```python
from build123d import *

# Parameters (mm, degrees)
BOSS_EXTRUDE1_DEPTH = 480


with BuildPart() as part:
    # Sketch1 → Boss-Extrude1 (new body)
    with BuildSketch(Plane(origin=(0, 0, 0), x_dir=(1, 0, 0), z_dir=(0, 1, 0))):
        with BuildLine():
            Line((20, 5.42), (20, 0.5))
            ThreePointArc((20, 0.5), (19.853553391, 0.146446609), (19.5, 0))
            Line((19.5, 0), (14.58, 0))
            Line((14.58, 0), (13.13, 1.549339828))
            Line((13.13, 1.549339828), (13.13, 1.799339828))
            Line((13.13, 1.799339828), (15.5, 1.799339828))
            Line((15.5, 1.799339828), (15.5, 3.439339828))
            Line((15.5, 3.439339828), (12.84, 6.099339828))
            Line((12.84, 6.099339828), (10.25, 6.099339828))
            Line((10.25, 6.099339828), (10, 6.349339828))
            Line((10, 6.349339828), (9.75, 6.099339828))
            Line((9.75, 6.099339828), (7.16, 6.099339828))
            Line((7.16, 6.099339828), (4.5, 3.439339828))
            Line((4.5, 3.439339828), (4.5, 1.799339828))
            Line((4.5, 1.799339828), (6.875, 1.799339828))
            Line((6.875, 1.799339828), (6.875, 1.549339828))
            Line((6.875, 1.549339828), (5.42, 0))
            Line((5.42, 0), (0.5, 0))
            ThreePointArc((0.5, 0), (0.146446609, 0.146446609), (0, 0.5))
            Line((0, 0.5), (0, 5.42))
            Line((0, 5.42), (1.549339828, 6.87))
            Line((1.549339828, 6.87), (1.799339828, 6.87))
            Line((1.799339828, 6.87), (1.799339828, 4.5))
            Line((1.799339828, 4.5), (3.439339828, 4.5))
            Line((3.439339828, 4.5), (6.099339828, 7.16))
            Line((6.099339828, 7.16), (6.099339828, 9.75))
            Line((6.099339828, 9.75), (6.349339828, 10))
            Line((6.349339828, 10), (6.099339828, 10.25))
            Line((6.099339828, 10.25), (6.099339828, 12.84))
            Line((6.099339828, 12.84), (3.439339828, 15.5))
            Line((3.439339828, 15.5), (1.799339828, 15.5))
            Line((1.799339828, 15.5), (1.799339828, 13.125))
            Line((1.799339828, 13.125), (1.549339828, 13.125))
            Line((1.549339828, 13.125), (0, 14.58))
            Line((0, 14.58), (0, 19.5))
            ThreePointArc((0, 19.5), (0.146446609, 19.853553391), (0.5, 20))
            Line((0.5, 20), (5.42, 20))
            Line((5.42, 20), (6.87, 18.450660172))
            Line((6.87, 18.450660172), (6.87, 18.200660172))
            Line((6.87, 18.200660172), (4.5, 18.200660172))
            Line((4.5, 18.200660172), (4.5, 16.560660172))
            Line((4.5, 16.560660172), (7.16, 13.900660172))
            Line((7.16, 13.900660172), (9.75, 13.900660172))
            Line((9.75, 13.900660172), (10, 13.650660172))
            Line((10, 13.650660172), (10.25, 13.900660172))
            Line((10.25, 13.900660172), (12.84, 13.900660172))
            Line((12.84, 13.900660172), (15.5, 16.560660172))
            Line((15.5, 16.560660172), (15.5, 18.200660172))
            Line((15.5, 18.200660172), (13.125, 18.200660172))
            Line((13.125, 18.200660172), (13.125, 18.450660172))
            Line((13.125, 18.450660172), (14.58, 20))
            Line((14.58, 20), (19.5, 20))
            ThreePointArc((19.5, 20), (19.853553391, 19.853553391), (20, 19.5))
            Line((20, 19.5), (20, 14.58))
            Line((20, 14.58), (18.450660172, 13.13))
            Line((18.450660172, 13.13), (18.200660172, 13.13))
            Line((18.200660172, 13.13), (18.200660172, 15.5))
            Line((18.200660172, 15.5), (16.560660172, 15.5))
            Line((16.560660172, 15.5), (13.900660172, 12.84))
            Line((13.900660172, 12.84), (13.900660172, 10.25))
            Line((13.900660172, 10.25), (13.650660172, 10))
            Line((13.650660172, 10), (13.900660172, 9.75))
            Line((13.900660172, 9.75), (13.900660172, 7.16))
            Line((13.900660172, 7.16), (16.560660172, 4.5))
            Line((16.560660172, 4.5), (18.200660172, 4.5))
            Line((18.200660172, 4.5), (18.200660172, 6.875))
            Line((18.200660172, 6.875), (18.450660172, 6.875))
            Line((18.450660172, 6.875), (20, 5.42))
        make_face()
        with BuildLine():
            ThreePointArc((12.1, 10), (11.48492424, 11.48492424), (10, 12.1))
            ThreePointArc((10, 12.1), (8.51507576, 11.48492424), (7.9, 10))
            ThreePointArc((7.9, 10), (8.51507576, 8.51507576), (10, 7.9))
            ThreePointArc((10, 7.9), (11.48492424, 8.51507576), (12.1, 10))
        make_face(mode=Mode.SUBTRACT)
    extrude(amount=BOSS_EXTRUDE1_DEPTH)


solid = part.part
```
Input: part model. Units: mm. Frame: model coordinates. Coordinates: 2 decimals unless noted, no trailing zeros. Use a Markdown table: item, result. Add a question column.
1) Draft query along Y for faces 1 (the flat face through (12.4, 480, -10.1)), 2 (the flat face through (12.4, 0, -10.1)). Return one class per face: +Y half, -Y half, draft (parallel to the pull), parting line (faces both ways), or undercut.
2) Pin query (flat end, axial travel): P1, Ø5, axis at x = 8.5, y = 313.5, coming from the -Z side; P2, Ø2, axis at y = 326.5, z = -7.5, coming from the +X side; P3, Ø2, axis at y = 162, z = -11.5, coming from the -X side. Return the tip coordinate at first contact, or that it passes through.
3) Line query: L1, parallel to X at y = 406, z = -3; L2, parallel to Z at x = 18, y = 240; L3, parallel to X at y = 411, z = -14. Output: solid intervals per line, ascending. Write a range as from..to.
Answer below:
| question | item | result |
|---|---|---|
| 1 | face 1 | +Y half |
| 1 | face 2 | -Y half |
| 2 | P1 | z = -19.38 |
| 2 | P2 | x = 18.85 |
| 2 | P3 | x = 6.1 |
| 3 | L1 | 0..4.5, 15.5..20 |
| 3 | L2 | -20..-15.5, -4.5..0 |
| 3 | L3 | 0.62..1.8, 4.94..7.06, 12.94..15.06, 18.2..19.38 |
